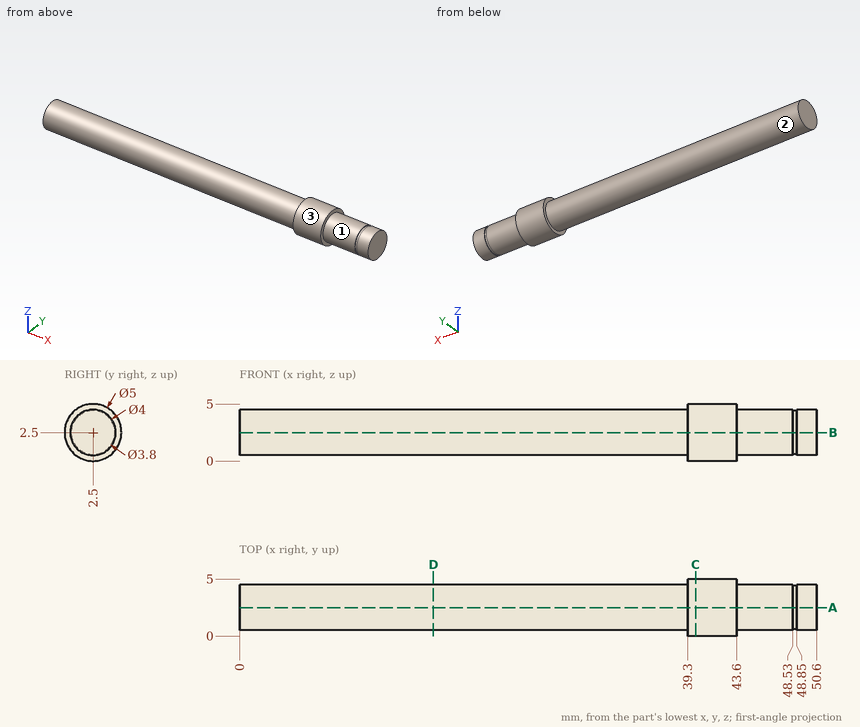
Geometry check sheet. Reference: drawing and pictorial views, mm from the part's lowest x, y, z. A direction names the side the tool comes from. Give positions to 0.01 mm unless a question says otherwise; leave off trailing zeros. Write each loop counter-clockwise with the first axis right and the second up, starting at its lowest first coordinate (ties: lowest second). Pieces come first, ordered by that corner, then holes. Notation, with made-up numbers: (68.5, 89.25) -> (103.5, 89.25) arc R25 ccw to (103.5, 108.25) -> close; hole circle Ø1 at (56, 24.5). An arc over 180 degrees is marked (long way). One line per item, written item: value. Start each with the question number.
Item 1: Section check C-C on x = 40. Record the cut outline in (y, z).
Item 2: Section check A-A on y = 2.5. Record the cut outline in (x, z), then the cut area to 3 significant figures.
Item 3: Material ranges on probe 1 along Z at (x, y) = (12.5, 2.45); probe 2 along Y at (x, z) = (11.5, 3.1), recorded low to high. Write a range as from..to.
Item 4: Gauge pin test, flat ends, axial feed: pin 1 (1 mm diameter, centred on x = 38.5, y = 1.5, fed in from -Z); pin 2 (2 mm diameter, centred on x = 20, z = 4, fed in from -Y); pin 3 (2 mm diameter, centred on x = 22.5, y = 0.5, fed in from +Z). Record the tip position at first contact, or that the pin passes through.
Item 5: Tool access check on the marked faces 1, 2 and 3. Record the directions out of +Z, -Z, +X, -X, +Y, -Y that give a thin tool (end or side, any length) a straight path to the whole face; none if there is none.
Item 6: Section check D-D on x = 17. Record the cut outline in (y, z).
Results list:
1. outline: circle Ø5 at (2.5, 2.5)
2. outline: (0, 0.5) -> (39.3, 0.5) -> (39.3, 0) -> (43.6, 0) -> (43.6, 0.5) -> (48.53, 0.5) -> (48.53, 0.6) -> (48.85, 0.6) -> (48.85, 0.5) -> (50.6, 0.5) -> (50.6, 4.5) -> (48.85, 4.5) -> (48.85, 4.4) -> (48.53, 4.4) -> (48.53, 4.5) -> (43.6, 4.5) -> (43.6, 5) -> (39.3, 5) -> (39.3, 4.5) -> (0, 4.5) -> close
2. area: 207 mm²
3. probe 1: 0.5..4.5
3. probe 2: 0.59..4.41
4. pin 1: z = 0.56
4. pin 2: y = 0.56
4. pin 3: z = 4.23
5. face 1: +X
5. face 2: -X
5. face 3: +X, -X
6. outline: circle Ø4 at (2.5, 2.5)
